```python
from build123d import *
from build123d.topology import SkipClean

# Parameters (mm, degrees)
SKETCH_1_W               = 16
SKETCH_1_H               = 16
SKETCH_1_R               = 1.55
EXTRUDE_1_DEPTH          = 3
SWEEP_1_PITCH            = 3
CUT_EXTRUDE_2_DEPTH      = 13.033723282
CUT_EXTRUDE_2_DEPTH_BACK = 13.033723282
SKETCH_8_R               = 0.6
CUT_EXTRUDE_3_DEPTH      = 12.704700005
SKETCH_11_W              = 16
SKETCH_11_H              = 6
SKETCH_11_R              = 0.6
EXTRUDE_2_DEPTH          = 0.4


with BuildPart() as part:
    # 草图1 → 凸台-拉伸1 (new, symmetric)
    with BuildSketch(Plane.XY):
        Rectangle(SKETCH_1_W, SKETCH_1_H)
        Circle(SKETCH_1_R, mode=Mode.SUBTRACT)
    extrude(amount=EXTRUDE_1_DEPTH, both=True)

    # 扫描1: arcs per turn and ends read off the stored shape
    # 扫描1: the profile of 草图10 profile screwed along a left-hand helix through 2 turns, 10 arcs to a turn; built about Z, then put on its axis
    sweep_1_z = Axis((0, 0, 0), (0, 0, 1))
    sweep_1_corners = [(1.5503, 0, -0.39994), (1.5503, 0, -1.10006), (1.05, 0, -1), (1.05, 0, -0.5)]
    with BuildLine(mode=Mode.PRIVATE) as sweep_1_profile:
        Line(sweep_1_corners[0], sweep_1_corners[1])
        Line(sweep_1_corners[1], sweep_1_corners[2])
        Line(sweep_1_corners[2], sweep_1_corners[3])
        Line(sweep_1_corners[3], sweep_1_corners[0])
    sweep_1_cap = Face(sweep_1_profile.wire())
    sweep_1_turn_angles = [0, -18, -36, -54, -72, -90, -108, -126, -144, -162, -180, -198, -216, -234, -252, -270, -288, -306, -324, -342, -360]
    sweep_1_turn_weights = [1, 0.9510565162951535, 1, 0.9510565162951535, 1, 0.9510565162951535, 1, 0.9510565162951535, 1, 0.9510565162951535, 1, 0.9510565162951535, 1, 0.9510565162951535, 1, 0.9510565162951535, 1, 0.9510565162951535, 1, 0.9510565162951535, 1]
    sweep_1_turn_rails = [Edge.make_bspline([Vector(p[0], p[1], 0).rotate(sweep_1_z, sweep_1_turn_angles[k]) / sweep_1_turn_weights[k] + Vector(0, 0, p[2] + -SWEEP_1_PITCH * sweep_1_turn_angles[k] / 360) for k in range(21)], [0, 0, 0, 1, 1, 2, 2, 3, 3, 4, 4, 5, 5, 6, 6, 7, 7, 8, 8, 9, 9, 10, 10, 10], 2, sweep_1_turn_weights) for p in sweep_1_corners]
    sweep_1_turn_sides = [Face.make_surface_from_curves(sweep_1_turn_rails[p[0]], sweep_1_turn_rails[p[1]]) for p in [(0, 1), (1, 2), (2, 3), (3, 0)]]
    sweep_1 = Plane(origin=(0, 0, 3), x_dir=(1, 0, 0), z_dir=(0, 0, -1)) * Solid(Shell([*[p.moved(Location((0, 0, SWEEP_1_PITCH * i))) for i in range(2) for p in sweep_1_turn_sides], sweep_1_cap, sweep_1_cap.rotate(sweep_1_z, -720).moved(Location((0, 0, -SWEEP_1_PITCH * -720 / 360)))]))
    add(sweep_1)

    # 草图7 → 切除-拉伸2 (cut, two sides: drawn at the far end of the back side and taken through both)
    with BuildSketch(Plane.XY.offset(-CUT_EXTRUDE_2_DEPTH_BACK)):
        with BuildLine():
            Line((-8, -0.271759997), (-1.014222118, -0.271759997))
            ThreePointArc((-1.014222118, -0.271759997), (-0.137052502, 1.041017104), (1.05, 0))
            ThreePointArc((1.05, 0), (1.041017104, -0.137052502), (1.014222118, -0.271759997))
            Line((1.014222118, -0.271759997), (8, -0.271759997))
            Line((8, -0.271759997), (8, 8))
            Line((8, 8), (-8, 8))
            Line((-8, 8), (-8, -0.271759997))
        make_face()
        with BuildLine():
            Line((1.014222118, -0.271759997), (0, 0))
            Line((0, 0), (-1.014222118, -0.271759997))
            ThreePointArc((-1.014222118, -0.271759997), (0, -1.05), (1.014222118, -0.271759997))
        make_face()
        with BuildLine():
            Line((-1.014222118, -0.271759997), (0, 0))
            Line((0, 0), (1.014222118, -0.271759997))
            ThreePointArc((1.014222118, -0.271759997), (1.041017104, -0.137052502), (1.05, 0))
            ThreePointArc((1.05, 0), (-0.137052502, 1.041017104), (-1.014222118, -0.271759997))
        make_face()
    extrude(amount=CUT_EXTRUDE_2_DEPTH + CUT_EXTRUDE_2_DEPTH_BACK, mode=Mode.SUBTRACT)

    # 草图8 → 切除-拉伸3 (cut, through all)
    with BuildSketch(Plane(origin=(0, 0, 0), x_dir=(1, 0, 0), z_dir=(0, 1, 0))):
        with Locations(Location((-5, 0, 0), (0, 0, 270))):
            Circle(SKETCH_8_R)
        with Locations(Location((5, 0, 0), (0, 0, 270))):
            Circle(SKETCH_8_R)
    extrude(amount=-CUT_EXTRUDE_3_DEPTH, mode=Mode.SUBTRACT)

    # 草图11 → 凸台-拉伸2 (add)
    with SkipClean():  # the faces are left unmerged after this step: merging them gives an invalid solid
        with BuildSketch(Plane.XZ.offset(8)):
            Rectangle(SKETCH_11_W, SKETCH_11_H)
            with Locations((5, 0)):
                Circle(SKETCH_11_R, mode=Mode.SUBTRACT)
            with Locations(Location((-5, 0, 0), (0, 0, 180))):
                Circle(SKETCH_11_R, mode=Mode.SUBTRACT)
        extrude(amount=EXTRUDE_2_DEPTH)


solid = part.part
```
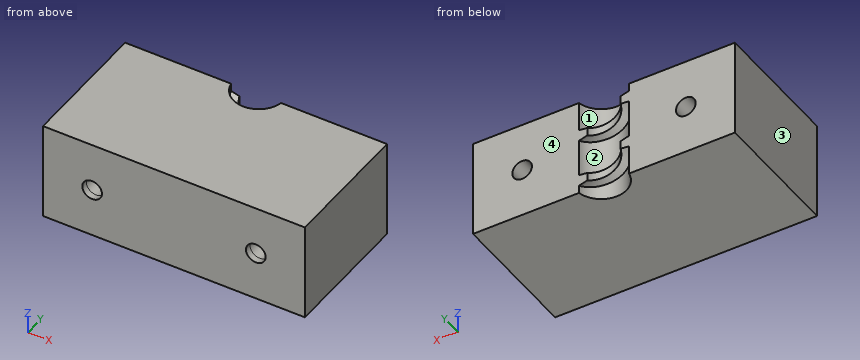
Build history of the part. All positions in model axes, mm. Face numbers are marked on the shaded views. Give positions to 0.01 mm unless a question says otherwise; leave off trailing zeros. Loops run counter-clockwise (first coordinate to the right, second up) from the corner with the lowest first, then second, coordinate; pieces in that order, holes last. Notation, with made-up numbers: (32, 63.25) - (82, 63.25) arc R22 cw to (82, 98.25) - close; hole circle Ø11 at (-10.75, 63). An arc over 180 degrees is marked (long way). Use a Markdown table: item, result.
(1) Wall check: line 1 along X through (y, z) = (-2.5, 0); line 2 along X through (y, z) = (-1.25, -0.5); line 3 along X through (y, z) = (-1, 2.5). Give the ranges that are in metal, low to high.
Taken from the geometry:
| item | result |
|---|---|
| line 1 | -8 to -5.6, -4.4 to 4.4, 5.6 to 8 |
| line 2 | -8 to -5.33, -4.67 to -0.92, 0.92 to 4.67, 5.33 to 8 |
| line 3 | -8 to -1.18, 1.18 to 8 |
(2) Pull direction X, two halves, no side cores. Call the marked faces 1, 2, 3 and 4: +X half, -X half, draft (parallel to the pull), parting line (faces both ways), or undercut.
Taken from the geometry:
| item | result |
|---|---|
| face 1 | undercut |
| face 2 | undercut |
| face 3 | -X half |
| face 4 | draft |
(3) Band-saw the part on B-B (x = -5). Give the cut face in (y, z), and give its area (3 significant figures).
Taken from the geometry:
| item | result |
|---|---|
| outline | (-8.4, -3) - (-0.27, -3) - (-0.27, -0.6) - (-8.4, -0.6) - close; (-8.4, 0.6) - (-0.27, 0.6) - (-0.27, 3) - (-8.4, 3) - close |
| area | 39.0 mm2 |
(4) Band-saw the part on C-C (y = -3.25). Give the cut face in (x, z).
Taken from the geometry:
| item | result |
|---|---|
| outline | (-8, -3) - (8, -3) - (8, 3) - (-8, 3) - close; hole circle Ø1.2 at (-5, 0); hole circle Ø1.2 at (5, 0) |
(5) Band-saw the part on A-A (z = 0). Give the cut face in (x, y), and give its area (3 significant figures).
Taken from the geometry:
| item | result |
|---|---|
| outline | (-8, -8.4) - (-5.6, -8.4) - (-5.6, -0.27) - (-8, -0.27) - close; (-4.4, -8.4) - (4.4, -8.4) - (4.4, -0.27) - (1.53, -0.27) arc R1.55 cw to (-1.53, -0.27) - (-4.4, -0.27) - close; (5.6, -8.4) - (8, -8.4) - (8, -0.27) - (5.6, -0.27) - close |
| area | 108 mm2 |
(6) Drop a flat-ended pin along its axis: pin 1 Ø0.7 at (x, z) = (-5, 0) entering from +Y. Give the stop position or say it passes through.
Taken from the geometry:
| item | result |
|---|---|
| pin 1 | through |
